from build123d import *

# Parameters (mm, degrees)
SKETCH2_R           = 2
EXTRUDE1_DEPTH      = 6
EXTRUDE1_DEPTH_BACK = 6
SKETCH3_R           = 2
EXTRUDE2_DEPTH      = 0.6
EXTRUDE2_TAPER      = 15
SKETCH4_R           = 2
EXTRUDE3_DEPTH      = 0.6
EXTRUDE3_TAPER      = 15


with BuildPart() as part:
    # Sketch2 → Extrude1 (new body, two sides)
    with BuildSketch(Plane(origin=(0, 0, 0), x_dir=(0, 0, -1), z_dir=(1, 0, 0))) as extrude1_sk:
        Circle(SKETCH2_R)
    extrude(amount=EXTRUDE1_DEPTH)
    extrude(extrude1_sk.sketch, amount=-EXTRUDE1_DEPTH_BACK)

    # Sketch3 → Extrude2 (add)
    with BuildSketch(Plane(origin=(6, 0, 0), x_dir=(0, 0, -1), z_dir=(1, 0, 0))):
        Circle(SKETCH3_R)
    extrude(amount=EXTRUDE2_DEPTH, taper=EXTRUDE2_TAPER)

    # Sketch4 → Extrude3 (add)
    with BuildSketch(Plane.ZY.offset(6)):
        Circle(SKETCH4_R)
    extrude(amount=EXTRUDE3_DEPTH, taper=EXTRUDE3_TAPER)


solid = part.part
Can you work these out from the model? Positions are in its coordinate system, mm. Give positions to 0.01 mm unless a question says otherwise; leave off trailing zeros. Order: outer loops, then holes, each group sorted by start corner. A loop starts at its lowest first (then second) coordinate and runs counter-clockwise, first axis right, second up. Notation, with made-up numbers: M 0.25,48 L 27.25,48 A18 cw 27.25,59 Z; hole C 39,40 d3. An arc over 180 degrees is marked long. Use one line per item in the form item = value. Start each with the question number.
Item 1: If I drill on line 1 along Z through (x, y) = (-1.5, -1.15); line 2 along Y through (x, z) = (4.25, 0.2); line 3 along Z through (x, y) = (-3, 1.8), over which ranges is the centre line in solid material (lowest first)?
Item 2: If we section it at A-A (x = 0.75): Write out the boundary of the cut face in (y, z), then the cut area to 3 significant figures.
Item 3: Will these pins go through, and if not, where does the flat tip stop? pin 1 Ø1 at (x, y) = (-1.5, -1) entering from +Z; pin 2 Ø1.5 at (x, z) = (3, 1.5) entering from -Y; pin 3 Ø2 at (x, y) = (-2, 1.5) entering from -Z.
Outcome:
q1.line_1 = -1.64 to 1.64
q1.line_2 = -1.99 to 1.99
q1.line_3 = -0.87 to 0.87
q2.outline = C 0,0 d4
q2.area = 12.6 mm2
q3.pin_1 = 1.94
q3.pin_2 = -1.85
q3.pin_3 = -1.94
